Part model, mm, in its own coordinate system. A direction names the side the tool comes from. Round coordinates to 2 decimals unless told otherwise and drop trailing zeros. Write each loop counter-clockwise with the first axis right and the second up, starting at its lowest first coordinate (ties: lowest second). Pieces come first, ordered by that corner, then holes.
```python
from build123d import *

# Parameters (mm, degrees)
F1_DEPTH = 20
F2_R     = 4
F2_R_2   = 1.5
F3_DEPTH = 4
F4_DEPTH = 25


with BuildPart() as f1:
    # F0 (on Top) → F1 (new body)
    with BuildSketch(Plane.XY):
        with BuildLine():
            ThreePointArc((4.9580672995, -35.5026810684), (12.8277785568, -32.8128229291), (19.6104349345, -28))
            ThreePointArc((19.6104349345, -28), (13.8230470925, -23.7215179323), (7.1602693698, -21))
            Line((7.1602693698, -21), (-7.9393995008, -21))
            ThreePointArc((-7.9393995008, -21), (-14.6021772235, -23.7215179323), (-20.3895650655, -28))
            ThreePointArc((-20.3895650655, -28), (-13.6069086879, -32.8128229291), (-5.7371974305, -35.5026810684))
            Line((-5.7371974305, -35.5026810684), (-0.3895650655, -34.5))
            Line((-0.3895650655, -34.5), (4.9580672995, -35.5026810684))
        make_face()
        with BuildLine():
            ThreePointArc((17.3657158391, -28), (9.0642701351, -32.8239230172), (-0.3895650655, -34.5))
            ThreePointArc((-0.3895650655, -34.5), (-9.8434002661, -32.8239230172), (-18.1448459701, -28))
            ThreePointArc((-18.1448459701, -28), (-0.3895650655, -21.5), (17.3657158391, -28))
        make_face(mode=Mode.SUBTRACT)
        with BuildLine():
            Line((7.6104349345, -36), (4.9580672995, -35.5026810684))
            ThreePointArc((4.9580672995, -35.5026810684), (2.295788637, -35.8754026031), (-0.3895650655, -36))
            Line((-0.3895650655, -36), (7.6104349345, -36))
        make_face()
        with BuildLine():
            Line((-8.3895650655, -36), (-0.3895650655, -36))
            ThreePointArc((-0.3895650655, -36), (-3.074918768, -35.8754026031), (-5.7371974305, -35.5026810684))
            Line((-5.7371974305, -35.5026810684), (-8.3895650655, -36))
        make_face()
        with BuildLine():
            ThreePointArc((-0.3895650655, -36), (2.295788637, -35.8754026031), (4.9580672995, -35.5026810684))
            Line((4.9580672995, -35.5026810684), (-0.3895650655, -34.5))
            Line((-0.3895650655, -34.5), (-5.7371974305, -35.5026810684))
            ThreePointArc((-5.7371974305, -35.5026810684), (-3.074918768, -35.8754026031), (-0.3895650655, -36))
        make_face()
        with BuildLine():
            Line((-7.9393995008, -21), (7.1602693698, -21))
            ThreePointArc((7.1602693698, -21), (-0.3895650655, -20), (-7.9393995008, -21))
        make_face()
        with BuildLine():
            ThreePointArc((-7.9393995008, -21), (-0.3895650655, -20), (7.1602693698, -21))
            Line((7.1602693698, -21), (21, -21))
            Line((21, -21), (21, -18))
            Line((21, -18), (0, -18))
            Line((0, -18), (-21, -18))
            Line((-21, -18), (-21, -21))
            Line((-21, -21), (-7.9393995008, -21))
        make_face()
    extrude(amount=F1_DEPTH)

    # F2 (on face) → F3 (cut)
    with BuildSketch(Plane.XZ.offset(36)):
        with Locations((-0.3895650655, 10)):
            Circle(F2_R)
        with Locations((-0.3895650655, 10)):
            Circle(F2_R_2, mode=Mode.SUBTRACT)
    extrude(amount=-F3_DEPTH, mode=Mode.SUBTRACT)

    # F4 (cut): a face of the model
    f4_faces = [f1.faces().sort_by_distance(p)[0] for p in [
        (-0.3895650655, -36, 10),
    ]]
    extrude(f4_faces, amount=-F4_DEPTH, mode=Mode.SUBTRACT)


solid = f1.part
```
Q1. Cut at C-C on x = -6.5. Write the cut outline in (y, z), plus the area to 3 significant figures.
Values follow:
outline: (-36, 0) - (-35.65, 0) - (-35.65, 20) - (-36, 20) - close; (-35.35, 0) - (-33.81, 0) - (-33.81, 20) - (-35.35, 20) - close; (-22.19, 0) - (-18, 0) - (-18, 20) - (-22.19, 20) - close
area: 122 mm2
Q2. Drop flat-ended pins along their axis: pin 1 (1.5 mm diameter, centred on y = -29.5, z = 13.5, fed in from -X); pin 2 (2 mm diameter, centred on y = -22.5, z = 17, fed in from -X); pin 3 (4 mm diameter, centred on x = -16, z = 8, fed in from -Y). Give the stop position or say it passes through.
Values follow:
pin 1: stops at x = -19.57
pin 2: stops at x = -14.2
pin 3: stops at y = -32.61
Q3. Cut at D-D on z = 17. Write the cut outline in (x, y), plus the area to 3 significant figures.
Values follow:
outline: (-21, -21) - (-7.94, -21) arc R29 ccw to (-20.39, -28) arc R29 ccw to (-5.74, -35.5) - (-8.39, -36) - (7.61, -36) - (4.96, -35.5) arc R29 ccw to (19.61, -28) arc R29 ccw to (7.16, -21) - (21, -21) - (21, -18) - (-21, -18) - close; hole (-18.14, -28) arc R27.5 ccw to (17.37, -28) arc R27.5 ccw to start
area: 243 mm2
Q4. Cut at B-B on y = -23. Write the cut outline in (x, z), plus the area to 3 significant figures.
Values follow:
outline: (-13.23, 0) - (-9.35, 0) - (-9.35, 20) - (-13.23, 20) - close; (8.57, 0) - (12.46, 0) - (12.46, 20) - (8.57, 20) - close
area: 155 mm2
Q5. Mould opens along Z. For faces 6 (the flat face through (-15, -21, 10)), 7 (the flat face through (0, -21, 20)), 8 (the cylindrical face through (-0.715, -19.796, 8.536)) say: +Z half, -Z half, draft (parallel to the pull), parting line (faces both ways), or undercut.
Values follow:
face 6: draft
face 7: +Z half
face 8: undercut
Q6. Cut at A-A on z = 10. Write the cut outline in (x, y), plus the area to 3 significant figures.
Values follow:
outline: (-21, -21) - (-7.94, -21) arc R29 ccw to (-20.39, -28) arc R29 ccw to (-5.74, -35.5) - (-8.39, -36) - (-4.39, -36) - (-4.39, -34.21) arc R27.5 cw to (-18.14, -28) arc R27.5 cw to (-1.89, -21.54) - (-1.89, -18) - (-21, -18) - close; (1.11, -21.54) arc R27.5 cw to (17.37, -28) arc R27.5 cw to (3.61, -34.21) - (3.61, -36) - (7.61, -36) - (4.96, -35.5) arc R29 ccw to (19.61, -28) arc R29 ccw to (7.16, -21) - (21, -21) - (21, -18) - (1.11, -18) - close
area: 220 mm2
Q7. Which spindle directions (+Z, -Z, +X, -X, +Y, -Y) get a long thin tool onto all of the face, cutting with end or side? Do faces 1 (the flat face through (14, -21, 10)), 2 (the cylindrical face through (-0.7, -21.5, 12.1)), 3 (the flat face through (-21, -19, 10)), 4 (the flat face through (0, -21, 0)), 5 (the cylindrical face through (1.456, -35.116, 6.451)). Say none if no direction does.
Values follow:
face 1: +Z, -Z, +X
face 2: +Z, -Z
face 3: +Z, -Z, -X, +Y, -Y
face 4: -Z, +X, -X, +Y, -Y
face 5: -Y
Q8. Wall check: L1, parallel to X at y = -20.8, z = 10; L2, parallel to Y at x = 5.5, z = 3.25; L3, parallel to Y at x = -18, z = 17. Give the ranges that are in metal, low to high.
Values follow:
L1: x = -21 to -1.89, 1.11 to 21
L2: y = -36 to -35.6, -35.4 to -33.86, -22.14 to -18
L3: y = -30.04 to -28.12, -27.88 to -25.96, -21 to -18
